Design review of the part built by this model. Coordinates are the model's own, in mm. Round coordinates to 2 decimals unless told otherwise and drop trailing zeros. Loops run counter-clockwise (first coordinate to the right, second up) from the corner with the lowest first, then second, coordinate; pieces in that order, holes last. Notation, with made-up numbers: (28.5, 44) - (65.5, 44) arc R25 ccw to (65.5, 65) - close; hole circle Ø2 at (59.25, -34). An arc over 180 degrees is marked (long way). Return JSON: item names as keys, results as strings. Group by question number.
from build123d import *

# Parameters (mm, degrees)
SKETCH1_W               = 200
SKETCH1_H               = 15
FRONT_TOP_BEAM_DEPTH    = 18
SKETCH2_W               = 3.1
SKETCH2_H               = 15
FRONT_TOP_GROOVES_DEPTH = 16
FRONT_TOP_RIB_REACH     = 202.948
SKETCH3_W               = 5
SKETCH3_H               = 18


with BuildPart() as part:
    # Sketch1 → Front Top Beam (new body)
    with BuildSketch(Plane(origin=(0, 0, 0), x_dir=(1, 0, 0), z_dir=(0, 1, 0))):
        Rectangle(SKETCH1_W, SKETCH1_H)
    extrude(amount=FRONT_TOP_BEAM_DEPTH)

    # Sketch2 → Front Top Grooves (cut)
    with BuildSketch(Plane.XZ):
        with Locations((-96.05, 0)):
            Rectangle(SKETCH2_W, SKETCH2_H)
        with Locations((96.05, 0)):
            Rectangle(SKETCH2_W, SKETCH2_H)
    extrude(amount=-FRONT_TOP_GROOVES_DEPTH, mode=Mode.SUBTRACT)

    # Sketch3 → Front Top Rib (add, up to next)
    with BuildSketch(Plane(origin=(100, 0, 0), x_dir=(0, 0, -1), z_dir=(1, 0, 0)), mode=Mode.PRIVATE) as front_top_rib_sk1:
        with Locations((0, 9)):
            Rectangle(SKETCH3_W, SKETCH3_H)
    front_top_rib_tool1 = extrude(front_top_rib_sk1.sketch, amount=-FRONT_TOP_RIB_REACH, mode=Mode.PRIVATE) - part.part
    add(front_top_rib_tool1.solids().sort_by_distance((100, 9, 0))[0])
    add(front_top_rib_tool1.solids().sort_by_distance((100, 9, 0))[1])


solid = part.part
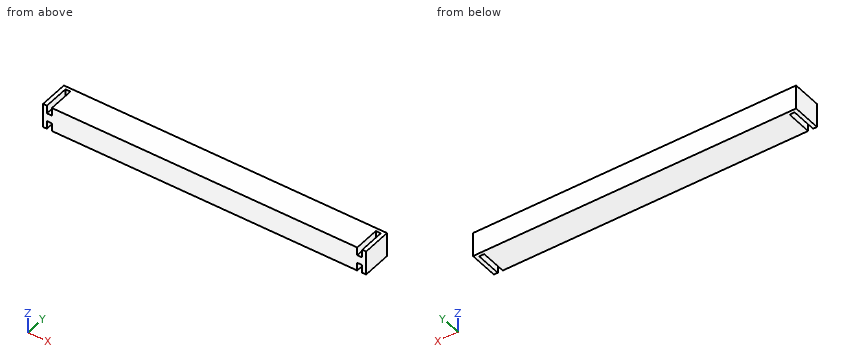
Q1. For line 1 (X direction, y = 4.75, z = -3.5), list the stretches that pass through material, from the lowest coordinate up.
Q2. Add section B-B, the plane y = 6. State the section outline as (x, z) points.
Q3. Add section A-A, the plane z = -5. State the section outline as (x, y) points.
Q4. Insertion check: pin 1 Ø0.9 at (x, y) = (95.5, 4.5) entering from -Z; pin 2 Ø1.5 at (x, z) = (96, 4.5) entering from -Y. Each pin has a flat end and moves straight along its axis. Give the tip position at first contact, or say it passes through.
Evaluation:
{
 "1": {"line 1": "-100 to -97.6, -94.5 to 94.5, 97.6 to 100"},
 "2": {"outline": "(-100, -7.5) - (-97.6, -7.5) - (-97.6, -2.5) - (-94.5, -2.5) - (-94.5, -7.5) - (94.5, -7.5) - (94.5, -2.5) - (97.6, -2.5) - (97.6, -7.5) - (100, -7.5) - (100, 7.5) - (97.6, 7.5) - (97.6, 2.5) - (94.5, 2.5) - (94.5, 7.5) - (-94.5, 7.5) - (-94.5, 2.5) - (-97.6, 2.5) - (-97.6, 7.5) - (-100, 7.5) - close"},
 "3": {"outline": "(-100, 0) - (-97.6, 0) - (-97.6, 16) - (-94.5, 16) - (-94.5, 0) - (94.5, 0) - (94.5, 16) - (97.6, 16) - (97.6, 0) - (100, 0) - (100, 18) - (-100, 18) - close"},
 "4": {"pin 1": "z = -2.5", "pin 2": "y = 16"}
}
